from build123d import *

# Parameters (mm, degrees)
SKETCH1_W           = 15
SKETCH1_H           = 28
BOSS_EXTRUDE1_DEPTH = 9.06
SKETCH2_R           = 1.4
CUT_EXTRUDE1_DEPTH  = 26
SKETCH3_W           = 2
SKETCH3_H           = 28
BOSS_EXTRUDE2_DEPTH = 85
CHAMFER1_SIZE       = 10
CHAMFER1_SIZE_2     = 43.314758743
SKETCH4_R           = 19.675
BOSS_EXTRUDE3_DEPTH = 2
CUT_EXTRUDE3_START  = -2
CUT_EXTRUDE3_DEPTH  = 2
FILLET1_R           = 20


with BuildPart() as part:
    # Sketch1 → Boss-Extrude1 (new body)
    with BuildSketch(Plane.XY):
        with Locations((7.5, 14)):
            Rectangle(SKETCH1_W, SKETCH1_H)
    extrude(amount=BOSS_EXTRUDE1_DEPTH)

    # Sketch2 → Cut-Extrude1 (cut)
    with BuildSketch(Plane.XY.offset(9.06)):
        with Locations((2.5, 24)):
            Circle(SKETCH2_R)
        with Locations((2.5, 19)):
            Circle(SKETCH2_R)
        with Locations((2.5, 9)):
            Circle(SKETCH2_R)
        with Locations((2.5, 4)):
            Circle(SKETCH2_R)
    extrude(amount=-CUT_EXTRUDE1_DEPTH, mode=Mode.SUBTRACT)

    # Sketch3 → Boss-Extrude2 (add)
    with BuildSketch(Plane(origin=(15, 0, 0), x_dir=(0, 0, -1), z_dir=(1, 0, 0))):
        with Locations((-8.06, 14)):
            Rectangle(SKETCH3_W, SKETCH3_H)
    extrude(amount=BOSS_EXTRUDE2_DEPTH)

    # Chamfer1
    # the kernel refuses this chamfer: 43.314758743, 10 mm, written as the material it adds along each edge
    with BuildSketch(Plane(origin=(15, 28, 7.06), x_dir=(-0.16038219639928503, 0, -0.9870549888826565), z_dir=(0, -1, 0))) as chamfer1_piece_1_section:
        Polygon((CHAMFER1_SIZE * 0.987054988883, CHAMFER1_SIZE * 0.160382196399), (-CHAMFER1_SIZE_2 * 0.160382196399, CHAMFER1_SIZE_2 * 0.987054988879), (0, 0), align=None)
    chamfer1_piece_1 = extrude(amount=28, mode=Mode.PRIVATE)
    chamfer1_piece_1 = split(chamfer1_piece_1, bisect_by=Plane(origin=(31.447908445, 14, 0), z_dir=(0, 0, 1)), keep=Keep.TOP, mode=Mode.PRIVATE)
    add(chamfer1_piece_1)

    # Sketch4 → Boss-Extrude3 (add)
    with BuildSketch(Plane.XY.offset(9.06)):
        with Locations((80.035, 14)):
            Circle(SKETCH4_R)
    extrude(amount=-BOSS_EXTRUDE3_DEPTH)

    # Sketch5 → Cut-Extrude3 (cut)
    with BuildSketch(Plane(origin=(0, 0, 7.06), x_dir=(-1, 0, 0), z_dir=(0, 0, -1)).offset(CUT_EXTRUDE3_START)):
        with BuildLine():
            ThreePointArc((-93.859095811, 0), (-99.71, 14), (-93.859095811, 28))
            Line((-93.859095811, 28), (-100, 28))
            Line((-100, 28), (-100, 0))
            Line((-100, 0), (-93.859095811, 0))
        make_face()
    extrude(amount=CUT_EXTRUDE3_DEPTH, mode=Mode.SUBTRACT)

    # Fillet1
    fillet1_edges = [part.edges().sort_by_distance(p)[0] for p in [
        (58.314758743, 14, 7.06),
        (27.73453907, 14, 0),
    ]]
    fillet(fillet1_edges, radius=FILLET1_R)


solid = part.part
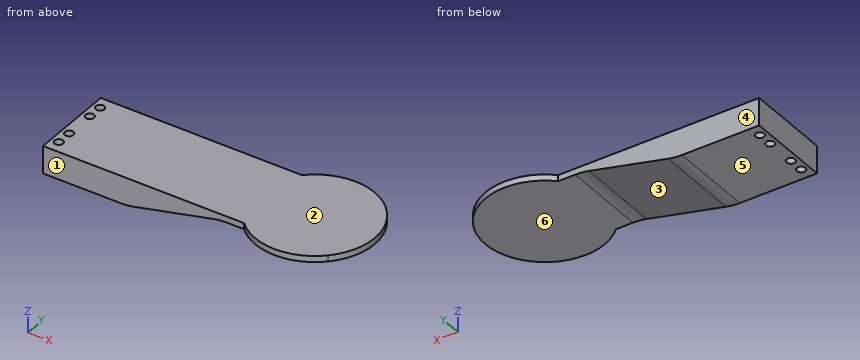
CAD build for the part. Positions are in the model's coordinates, mm. Face numbers are marked on the shaded views. A direction names the side the tool comes from. Coordinates: 2 decimals unless noted, no trailing zeros. Write each loop counter-clockwise with the first axis right and the second up, starting at its lowest first coordinate (ties: lowest second). Pieces come first, ordered by that corner, then holes. Notation, with made-up numbers: M 59,7 L 76,7 A26 cw 76,42 Z; hole C -39.75,-16.75 d10. An arc over 180 degrees is marked long. Return JSON: item names as keys, results as strings.
Item 1: Slice it at D-D, the plane y = 13. Write the cut outline in (x, z), and give its area (3 significant figures).
Findings below:
{"outline": "M 0,0 L 25.46,0 A20 ccw 29.95,0.51 L 56.09,6.55 A20 cw 60.59,7.06 L 99.68,7.06 L 99.68,9.06 L 0,9.06 Z", "area": "503 mm2"}
Item 2: Drop flat-ended pins along their axis: pin 1 Ø11.5 at (x, y) = (76.5, 15.5) entering from -Z; pin 2 Ø2 at (x, y) = (2.5, 4) entering from +Z; pin 3 Ø2.5 at (x, z) = (40.5, 5.5) entering from -Y; pin 4 Ø5 at (x, z) = (72.5, 6.5) entering from +Y. Give the stop position or say it passes through.
Findings below:
{"pin 1": "stops at z = 7.06", "pin 2": "passes through", "pin 3": "stops at y = 0", "pin 4": "stops at y = 33"}
Item 3: Which spindle directions (+Z, -Z, +X, -X, +Y, -Y) get a long thin tool onto all of the face, cutting with end or side? Do the marked faces 4, 5 and 6. Say none if no direction does.
Findings below:
{"face 4": "+Z, -Z, -X, +Y", "face 5": "-Z, +X, -X, +Y, -Y", "face 6": "-Z, +X, +Y, -Y"}
Item 4: Slice it at C-C, the plane z = 3.5. Write the cut outline in (x, y), and give its area (3 significant figures).
Findings below:
{"outline": "M 0,0 L 42.89,0 L 42.89,28 L 0,28 Z; hole C 2.5,4 d2.8; hole C 2.5,9 d2.8; hole C 2.5,19 d2.8; hole C 2.5,24 d2.8", "area": "1,180 mm2"}
Item 5: Slice it at B-B, the plane y = 24. Write the cut outline in (x, z), and give its area (3 significant figures).
Findings below:
{"outline": "M 0,0 L 1.1,0 L 1.1,9.06 L 0,9.06 Z; M 3.9,0 L 25.46,0 A20 ccw 29.95,0.51 L 56.09,6.55 A20 cw 60.59,7.06 L 96.98,7.06 L 96.98,9.06 L 3.9,9.06 Z", "area": "472 mm2"}
Item 6: Slice it at A-A, the plane x = 2.5. Write the cut outline in (y, z).
Findings below:
{"outline": "M 0,0 L 2.6,0 L 2.6,9.06 L 0,9.06 Z; M 5.4,0 L 7.6,0 L 7.6,9.06 L 5.4,9.06 Z; M 10.4,0 L 17.6,0 L 17.6,9.06 L 10.4,9.06 Z; M 20.4,0 L 22.6,0 L 22.6,9.06 L 20.4,9.06 Z; M 25.4,0 L 28,0 L 28,9.06 L 25.4,9.06 Z"}
Item 7: Two-plate mould, pull along Z, no slides. Class the marked faces 1, 2 and 3: +Z half, -Z half, draft (parallel to the pull), parting line (faces both ways), or undercut.
Findings below:
{"face 1": "draft", "face 2": "+Z half", "face 3": "-Z half"}
Item 8: Probe line 1 (Y direction, x = 2.5, z = 3.75); line 2 (Z direction, x = 71, y = 5.5); line 3 (Y direction, x = 35.5, z = 2.25). List the from-to ranges inside material, lowest first. Write a range as from..to.
Findings below:
{"line 1": "y = 0..2.6, 5.4..7.6, 10.4..17.6, 20.4..22.6, 25.4..28", "line 2": "z = 7.06..9.06", "line 3": "y = 0..28"}
